CAD build for the part. Positions are in the model's coordinates, mm. A direction names the side the tool comes from. Round coordinates to 2 decimals unless told otherwise and drop trailing zeros. Order: outer loops, then holes, each group sorted by start corner. A loop starts at its lowest first (then second) coordinate and runs counter-clockwise, first axis right, second up. Notation, with made-up numbers: M -38,39.25 L -5,39.25 A25 cw -5,54.25 Z; hole C 29.5,83 d7. An arc over 180 degrees is marked long. Answer as a JSON object with one key per item and string values. Group by question number.
```python
from build123d import *

# Parameters (mm, degrees)
F0_W     = 31.8
F0_H     = 15.8
F1_DEPTH = 9.6
F2_T     = -2.54
F3_R     = 3.043204
F4_DEPTH = 1.8


with BuildPart() as f1:
    # F0 (on Top) → F1 (new body)
    with BuildSketch(Plane.XY):
        with Locations((8.439594, 3.65301)):
            Rectangle(F0_W, F0_H)
    extrude(amount=-F1_DEPTH)

    # F2
    f2_openings = [f1.faces().sort_by_distance(p)[0] for p in [
        (8.439594, 3.65301, -9.6),
    ]]
    offset(amount=F2_T, openings=f2_openings)

    # F3 (on face) → F4 (join)
    with BuildSketch(Plane.XY):
        with Locations((19.01015, 8.054115)):
            Circle(F3_R)
        with Locations((19.01015, -0.545885)):
            Circle(F3_R)
        with Locations((8.01015, 8.054115)):
            Circle(F3_R)
        with Locations((8.01015, -0.545885)):
            Circle(F3_R)
        with Locations((-2.98985, 8.054115)):
            Circle(F3_R)
        with Locations((-2.98985, -0.545885)):
            Circle(F3_R)
    extrude(amount=F4_DEPTH)


solid = f1.part
```
Item 1: Cut at C-C, the plane y = 6. Give the cut face in (x, z).
Item 2: 3-axis set-ups, long thin cutter, end or side, ignore diameter. For faces 1 (the face through (8, 9.013, -6)), 2 (the face through (8, -4.247, -5)), 3 (the face through (10.913, 0.368, 0.887)): which of +Z, -Z, +X, -X, +Y, -Y reach the whole face in a straight line?
Item 3: Cut at A-A, the plane x = 4. Give the cut face in (y, z), and give its area (3 significant figures).
Item 4: Drill centre lines: line 1 (Y direction, x = 20.5, z = -5); line 2 (X direction, y = 2.5, z = -5.5); line 3 (Z direction, x = 7.5, y = 0). Where is each one in solid material? Low to high. Write a range as [from, to].
Item 5: Cut at D-D, the plane z = 0.5. Give the cut face in (x, y).
Item 6: Cut at B-B, the plane z = -7. Give the cut face in (x, y).
Item 7: Flat gauge pin, fed straight in: pin 1 Ø1.5 at (x, y) = (8, 0) entering from -Z. Where does the tip first touch, or does it go through?
Response values:
{
 "1": {"outline": "M -7.46,-9.6 L -4.92,-9.6 L -4.92,-2.54 L 21.8,-2.54 L 21.8,-9.6 L 24.34,-9.6 L 24.34,0 L 21.26,0 L 21.26,1.8 L 16.76,1.8 L 16.76,0 L 10.26,0 L 10.26,1.8 L 5.76,1.8 L 5.76,0 L -0.74,0 L -0.74,1.8 L -5.24,1.8 L -5.24,0 L -7.46,0 Z"},
 "2": {"face 1": "-Z", "face 2": "+Z, -Z, +X, -X, -Y", "face 3": "+Z"},
 "3": {"outline": "M -4.25,-9.6 L -1.71,-9.6 L -1.71,-2.54 L 9.01,-2.54 L 9.01,-9.6 L 11.55,-9.6 L 11.55,0 L -4.25,0 Z", "area": "76.0 mm^2"},
 "4": {"line 1": "[-4.25, -1.71], [9.01, 11.55]", "line 2": "[-7.46, -4.92], [21.8, 24.34]", "line 3": "[-2.54, 1.8]"},
 "5": {"outline": "C -2.99,-0.55 d6.09; C -2.99,8.05 d6.09; C 8.01,-0.55 d6.09; C 8.01,8.05 d6.09; C 19.01,-0.55 d6.09; C 19.01,8.05 d6.09"},
 "6": {"outline": "M -7.46,-4.25 L 24.34,-4.25 L 24.34,11.55 L -7.46,11.55 Z; hole M -4.92,-1.71 L 21.8,-1.71 L 21.8,9.01 L -4.92,9.01 Z"},
 "7": {"pin 1": "z = -2.54"}
}
